Build history of the part. All positions in model axes, mm. A direction names the side the tool comes from. Give positions to 0.01 mm unless a question says otherwise; leave off trailing zeros. Loops run counter-clockwise (first coordinate to the right, second up) from the corner with the lowest first, then second, coordinate; pieces in that order, holes last. Notation, with made-up numbers: M 37.25,55.25 L 67.25,55.25 A34 cw 67.25,87.25 Z; hole C 11,-37.75 d9. An arc over 180 degrees is marked long. Put each result on its own line as item: value.
```python
from build123d import *

# Parameters (mm, degrees)
EXTRUDE1_DEPTH                      = 12.7
EXTRUDE1_DEPTH_BACK                 = 12.7
F_6_CLEARANCE_HOLE1_D               = 3.7973
F_6_CLEARANCE_HOLE1_DEPTH           = 12.7
F_6_CLEARANCE_HOLE1_TIP             = 1.140824014
F_6_CLEARANCE_HOLE1_ON_FACE_2_D     = 3.7973
F_6_CLEARANCE_HOLE1_ON_FACE_2_DEPTH = 12.7
F_6_CLEARANCE_HOLE1_ON_FACE_2_TIP   = 1.140824014
SKETCH4_R                           = 11.43
CUT_EXTRUDE1_DEPTH                  = 4.175


with BuildPart() as part:
    # Sketch2 → Extrude1 (new body, two sides)
    with BuildSketch(Plane(origin=(0, 0, 0), x_dir=(0, 0, -1), z_dir=(1, 0, 0))) as extrude1_sk:
        Polygon((0, 0), (0, 12.7), (3.175, 12.7), (3.175, 3.175), (19.05, 3.175), (19.05, 0), align=None)
    extrude(amount=EXTRUDE1_DEPTH)
    extrude(extrude1_sk.sketch, amount=-EXTRUDE1_DEPTH_BACK)

    # 6 Clearance Hole1
    with Locations(Plane(origin=(6.35, 7.62, -3.175), x_dir=(0, -1, 0), z_dir=(0, 0, -1))):
        with Locations((0, 0), (0, 12.7)):
            Hole(F_6_CLEARANCE_HOLE1_D / 2, depth=F_6_CLEARANCE_HOLE1_DEPTH)
            with Locations((0, 0, -(F_6_CLEARANCE_HOLE1_DEPTH + F_6_CLEARANCE_HOLE1_TIP / 2))):  # 118° drill point
                Cone(0, F_6_CLEARANCE_HOLE1_D / 2, F_6_CLEARANCE_HOLE1_TIP, mode=Mode.SUBTRACT)

    # 6 Clearance Hole1 on face 2
    with Locations(Plane(origin=(6.35, 3.175, -12.7), x_dir=(0, 0, 1), z_dir=(0, 1, 0))):
        with Locations((0, 0), (0, -12.7)):
            Hole(F_6_CLEARANCE_HOLE1_ON_FACE_2_D / 2, depth=F_6_CLEARANCE_HOLE1_ON_FACE_2_DEPTH)
            with Locations((0, 0, -(F_6_CLEARANCE_HOLE1_ON_FACE_2_DEPTH + F_6_CLEARANCE_HOLE1_ON_FACE_2_TIP / 2))):  # 118° drill point
                Cone(0, F_6_CLEARANCE_HOLE1_ON_FACE_2_D / 2, F_6_CLEARANCE_HOLE1_ON_FACE_2_TIP, mode=Mode.SUBTRACT)

    # Sketch4 → Cut-Extrude1 (cut, through all)
    with BuildSketch(Plane(origin=(0, 0, -3.175), x_dir=(-1, 0, 0), z_dir=(0, 0, -1))):
        with Locations((0, 21.59)):
            Circle(SKETCH4_R)
    extrude(amount=-CUT_EXTRUDE1_DEPTH, mode=Mode.SUBTRACT)


solid = part.part
```
Q1. Probe line 1 (X direction, y = 1.8, z = -12.7); line 2 (Z direction, x = -5.5, y = 11.5) (3 decimals); line 3 (Y direction, x = 8.25, z = -11) (3 decimals). List the from-to ranges inside material, lowest first. Write a range as from..to.
Here are the results:
line 1: -12.7..-8.25, -4.45..4.45, 8.25..12.7
line 2: -3.175..0
line 3: 0..3.175
Q2. Slice it at B-B (y = 7.62). List the corners of the cut face in (x, z) (3 decimals), and give its area (3 significant figures).
Here are the results:
outline: M -12.7,-3.175 L -8.249,-3.175 L -8.249,0 L -12.7,0 Z; M -4.451,-3.175 L 4.451,-3.175 L 4.451,0 L -4.451,0 Z; M 8.249,-3.175 L 12.7,-3.175 L 12.7,0 L 8.249,0 Z
area: 56.5 mm²
Q3. Mould opens along Y. For faces 1 (the cylindrical face through (0.11, 10.16, -1.61)), 2 (the cylindrical face through (-4.666, 8.496, -1.565)), 3 (the flat face through (12.7, 3, -7)), 4 (the cylindrical face through (4.75, 8.64, -1.57)) say: pulls with the +Y half, pulls with the -Y half, needs draft (parallel to the pull), parting line crosses it, or undercut.
Here are the results:
face 1: pulls with the +Y half
face 2: undercut
face 3: needs draft
face 4: undercut
Q4. Slice it at D-D (y = 2.5). List the corners of the cut face in (x, z), and give its area (3 significant figures).
Here are the results:
outline: M -12.7,-19.05 L 12.7,-19.05 L 12.7,0 L -12.7,0 Z; hole C -6.35,-12.7 d3.8; hole C 6.35,-12.7 d3.8
area: 461 mm²
Q5. Tool access for faces 5 (the flat face through (0, 0, -10)), 6 (the flat face through (0, 8, -3.175)): list every direction of +Z, -Z, +X, -X, +Y, -Y with a clear straight run to the whole face (end or side of a thin tool).
Here are the results:
face 5: +Z, -Z, +X, -X, -Y
face 6: -Z, +X, -X, +Y
Q6. Slice it at A-A (z = -12.7). List the corners of the cut face in (x, y) (3 decimals), and give its area (3 significant figures).
Here are the results:
outline: M -12.7,0 L -8.249,0 L -8.249,3.175 L -12.7,3.175 Z; M -4.451,0 L 4.451,0 L 4.451,3.175 L -4.451,3.175 Z; M 8.249,0 L 12.7,0 L 12.7,3.175 L 8.249,3.175 Z
area: 56.5 mm²
Q7. Slice it at C-C (x = -6). List the corners of the cut face in (y, z) (3 decimals).
Here are the results:
outline: M 0,-19.05 L 3.175,-19.05 L 3.175,-14.566 L 0,-14.566 Z; M 0,-10.834 L 3.175,-10.834 L 3.175,-3.175 L 5.754,-3.175 L 5.754,0 L 0,0 Z; M 9.486,-3.175 L 11.861,-3.175 L 11.861,0 L 9.486,0 Z
Q8. Drop flat-ended pins along their axis: pin 1 Ø8 at (x, z) = (5, -14.5) entering from +Y (3 decimals); pin 2 Ø6 at (x, y) = (-6.35, 7.62) entering from -Z (3 decimals). Give the stop position or say it passes through.
Here are the results:
pin 1: y = 3.175
pin 2: z = -3.175
